Here's how the part is built. I have some questions about the finished solid (model axes, mm). Coordinates: 2 decimals unless noted, no trailing zeros. Write each loop counter-clockwise with the first axis right and the second up, starting at its lowest first coordinate (ties: lowest second). Pieces come first, ordered by that corner, then holes. Notation, with made-up numbers: (-38, 37.5) - (14, 37.5) arc R11 ccw to (14, 46.5) - close; hole circle Ø9 at (19, -33.5). An arc over 180 degrees is marked (long way). Answer in a Markdown table with one row per item. Add a question column.
Item 1: Imagine slicing it at C-C (z = 8). Please give me the cut outline in (x, y).
Item 2: I'm going to push a flat-ended pin straight in: pin 1 (2 mm diameter, centred on x = 17.5, z = 6, fed in from +Y). Where does the tip first touch, or does it pass through?
Item 3: Imagine slicing it at B-B (y = 68.25). Please give me the cut outline in (x, z).
Item 4: If I drill on probe 1 along Y at (x, z) = (15.75, 7.5); probe 2 along Y at (x, z) = (12.5, 8), over which ranges is the centre line in solid material (lowest first)? Write a range as from..to.
Item 5: Imagine slicing it at A-A (x = 6). Please give me the cut outline in (y, z).
from build123d import *

# Parameters (mm, degrees)
SKETCH015_W      = 18
SKETCH015_H      = 6.8
PAD006_DEPTH     = 8.5
CHAMFER002_SIZE2 = 1.4
CHAMFER002_SIZE  = 3.7
CHAMFER003_SIZE2 = 3.7
CHAMFER003_SIZE  = 1.4


with BuildPart() as part:
    # Sketch015 → Pad006 (new body)
    with BuildSketch(Plane.XY):
        with Locations((38.3, 65.1)):
            Rectangle(SKETCH015_W, SKETCH015_H)
    extrude(amount=PAD006_DEPTH)

    # Chamfer002
    chamfer002_edges = [part.edges().sort_by_distance(p)[0] for p in [
        (38.3, 68.5, 8.5),
    ]]
    chamfer002_side = part.faces().sort_by_distance((38.3, 68.5, 4.25))[0]
    chamfer(chamfer002_edges, length=CHAMFER002_SIZE, length2=CHAMFER002_SIZE2, reference=chamfer002_side)

    # Chamfer003
    chamfer003_edges = [part.edges().sort_by_distance(p)[0] for p in [
        (38.3, 61.7, 8.5),
    ]]
    chamfer003_side = part.faces().sort_by_distance((38.3, 64.4, 8.5))[0]
    chamfer(chamfer003_edges, length=CHAMFER003_SIZE, length2=CHAMFER003_SIZE2, reference=chamfer003_side)


with BuildPart() as part_1:
    # Body026 placement: moved
    add(part.part.moved(Location((-26.7, 0, 0))))


solid = part_1.part
Here are the results:
| question | item | result |
|---|---|---|
| 1 | outline | (2.6, 62.91) - (20.6, 62.91) - (20.6, 67.29) - (2.6, 67.29) - close |
| 2 | pin 1 | stops at y = 68.42 |
| 3 | outline | (2.6, 0) - (20.6, 0) - (20.6, 5.46) - (2.6, 5.46) - close |
| 4 | probe 1 | y = 62.72..67.48 |
| 4 | probe 2 | y = 62.91..67.29 |
| 5 | outline | (61.7, 0) - (68.5, 0) - (68.5, 4.8) - (67.1, 8.5) - (63.1, 8.5) - (61.7, 4.8) - close |
